The model under review builds one solid part; all positions refer to its coordinate system, in mm. A direction names the side the tool comes from. Round coordinates to 2 decimals unless told otherwise and drop trailing zeros. Order: outer loops, then holes, each group sorted by start corner. A loop starts at its lowest first (then second) coordinate and runs counter-clockwise, first axis right, second up.
from build123d import *

# Parameters (mm, degrees)
SKETCH_1_W                         = 50
SKETCH_1_H                         = 80
SM_BASE_FLANGE_1_DEPTH             = 3
SM_EDGE_FLANGE_1_STRIP_W           = 13.4732
SM_EDGE_FLANGE_1_STRIP_H           = 3
SM_EDGE_FLANGE_1_STRIP_CUT_DEPTH   = 50
SM_EDGE_FLANGE_1_STRIP_2_W         = 13.4732
SM_EDGE_FLANGE_1_STRIP_2_H         = 3
SM_EDGE_FLANGE_1_STRIP_CUT_2_DEPTH = 50
SM_EDGE_FLANGE_1_DEPTH             = 50
SM_EDGE_FLANGE_1_BEND_DEPTH        = 50
SM_EDGE_FLANGE_2_STRIP_W           = 13.4732
SM_EDGE_FLANGE_2_STRIP_H           = 3
SM_EDGE_FLANGE_2_STRIP_CUT_DEPTH   = 50
SM_EDGE_FLANGE_2_STRIP_2_W         = 13.4732
SM_EDGE_FLANGE_2_STRIP_2_H         = 3
SM_EDGE_FLANGE_2_STRIP_CUT_2_DEPTH = 50
SM_EDGE_FLANGE_2_DEPTH             = 50
SM_EDGE_FLANGE_2_BEND_DEPTH        = 50
SKETCH_18_R                        = 6.5
CUT_EXTRUDE_1_DEPTH                = 124


# Sheet-metal steps are written as plain solids
with BuildPart() as part:
    # Sketch 1 → 基体-法兰1 (new body)
    with BuildSketch(Plane.XY):
        with Locations((25, 40)):
            Rectangle(SKETCH_1_W, SKETCH_1_H)
    extrude(amount=-SM_BASE_FLANGE_1_DEPTH)

    # 边线-法兰1 strip (across the edge) → 边线-法兰1 strip cut (cut)
    with BuildSketch(Plane(origin=(0, 80, -3), x_dir=(0, -1, 0), z_dir=(1, 0, 0))):
        with Locations((-6, -1.5)):
            Rectangle(SM_EDGE_FLANGE_1_STRIP_W, SM_EDGE_FLANGE_1_STRIP_H)
    extrude(amount=SM_EDGE_FLANGE_1_STRIP_CUT_DEPTH, mode=Mode.SUBTRACT)

    # 边线-法兰1 strip 2 (across the edge) → 边线-法兰1 strip cut 2 (cut)
    with BuildSketch(Plane(origin=(50, 0, -3), x_dir=(0, 1, 0), z_dir=(-1, 0, 0))):
        with Locations((-6, -1.5)):
            Rectangle(SM_EDGE_FLANGE_1_STRIP_2_W, SM_EDGE_FLANGE_1_STRIP_2_H)
    extrude(amount=SM_EDGE_FLANGE_1_STRIP_CUT_2_DEPTH, mode=Mode.SUBTRACT)

    # 边线-法兰1 section (across the edge) → 边线-法兰1 (add)
    with BuildSketch(Plane(origin=(0, 80, -3), x_dir=(0, -1, 0), z_dir=(1, 0, 0))):
        with BuildLine():
            Line((-3, 0.7366), (-3, 17))
            Line((-3, 17), (0, 17))
            Line((0, 17), (0, 0.7366))
            ThreePointArc((0, 0.7366), (0.215745145, 0.215745145), (0.7366, 0))
            Line((0.7366, 0), (0.7366, -3))
            ThreePointArc((0.7366, -3), (-1.905575199, -1.905575199), (-3, 0.7366))
        make_face()
    extrude(amount=SM_EDGE_FLANGE_1_DEPTH)

    # 边线-法兰1 section 2 (across the edge) → 边线-法兰1 bend (add)
    with BuildSketch(Plane(origin=(50, 0, -3), x_dir=(0, 1, 0), z_dir=(-1, 0, 0))):
        with BuildLine():
            Line((-3, 0.7366), (-3, 17))
            Line((-3, 17), (0, 17))
            Line((0, 17), (0, 0.7366))
            ThreePointArc((0, 0.7366), (0.215745145, 0.215745145), (0.7366, 0))
            Line((0.7366, 0), (0.7366, -3))
            ThreePointArc((0.7366, -3), (-1.905575199, -1.905575199), (-3, 0.7366))
        make_face()
    extrude(amount=SM_EDGE_FLANGE_1_BEND_DEPTH)

    # 边线-法兰2 strip (across the edge) → 边线-法兰2 strip cut (cut)
    with BuildSketch(Plane(origin=(0, -3, -20), x_dir=(0, 0, 1), z_dir=(1, 0, 0))):
        with Locations((-6, -1.5)):
            Rectangle(SM_EDGE_FLANGE_2_STRIP_W, SM_EDGE_FLANGE_2_STRIP_H)
    extrude(amount=SM_EDGE_FLANGE_2_STRIP_CUT_DEPTH, mode=Mode.SUBTRACT)

    # 边线-法兰2 strip 2 (across the edge) → 边线-法兰2 strip cut 2 (cut)
    with BuildSketch(Plane(origin=(50, 83, -20), x_dir=(0, 0, 1), z_dir=(-1, 0, 0))):
        with Locations((-6, -1.5)):
            Rectangle(SM_EDGE_FLANGE_2_STRIP_2_W, SM_EDGE_FLANGE_2_STRIP_2_H)
    extrude(amount=SM_EDGE_FLANGE_2_STRIP_CUT_2_DEPTH, mode=Mode.SUBTRACT)

    # 边线-法兰2 section (across the edge) → 边线-法兰2 (add)
    with BuildSketch(Plane(origin=(0, -3, -20), x_dir=(0, 0, 1), z_dir=(1, 0, 0))):
        with BuildLine():
            Line((-3, 0.7366), (-3, 27))
            Line((-3, 27), (0, 27))
            Line((0, 27), (0, 0.7366))
            ThreePointArc((0, 0.7366), (0.215745145, 0.215745145), (0.7366, 0))
            Line((0.7366, 0), (0.7366, -3))
            ThreePointArc((0.7366, -3), (-1.905575199, -1.905575199), (-3, 0.7366))
        make_face()
    extrude(amount=SM_EDGE_FLANGE_2_DEPTH)

    # 边线-法兰2 section 2 (across the edge) → 边线-法兰2 bend (add)
    with BuildSketch(Plane(origin=(50, 83, -20), x_dir=(0, 0, 1), z_dir=(-1, 0, 0))):
        with BuildLine():
            Line((-3, 0.7366), (-3, 27))
            Line((-3, 27), (0, 27))
            Line((0, 27), (0, 0.7366))
            ThreePointArc((0, 0.7366), (0.215745145, 0.215745145), (0.7366, 0))
            Line((0.7366, 0), (0.7366, -3))
            ThreePointArc((0.7366, -3), (-1.905575199, -1.905575199), (-3, 0.7366))
        make_face()
    extrude(amount=SM_EDGE_FLANGE_2_BEND_DEPTH)

    # 草图18 → 切除-拉伸1 (cut, through all)
    with BuildSketch(Plane.XY):
        with Locations((25, 40)):
            Circle(SKETCH_18_R)
    extrude(amount=-CUT_EXTRUDE_1_DEPTH, mode=Mode.SUBTRACT)


solid = part.part
(1) To check wall thickness, follow L1, parallel to Y at x = 11.5, z = -15.5; L2, parallel to Z at x = 36.5, y = 6; L3, parallel to Z at x = 34.5, y = 91. State the ranges of each line that lie inside material, in increasing order.
(2) Tool access review of faces 1 (the flat face through (25, 83, -11)), 2 (the cylindrical face through (25.35, 81.07, -21.88)), 3 (the flat face through (25, 49, 0)): name each direction out of +Z, -Z, +X, -X, +Y, -Y from which nothing blocks a thin tool from reaching the whole face with its end or side.
(3) The part is to be moulded in two halves that separate along Y. For faces 4 (the flat face through (25, 110, -22)), 5 (the cylindrical face through (19.842, 36.045, -1.479)), 6 (the flat face through (25, -3, -11)), say which applies: pulls with the +Y half, pulls with the -Y half, needs draft (parallel to the pull), parting line crosses it, or undercut.
(4) We need section B-B (z = -10.5). Give the boundary of the cut face in (x, y), and give its area (3 significant figures).
(5) Clearance check with flat-ended pins moving along their axes: P1, Ø1.5, axis at x = 41, z = -13.5, coming from the -Y side; P2, Ø12.5, axis at x = 26, z = -14, coming from the +Y side; P3, Ø8, axis at x = 32, y = 22, coming from the -Z side; P4, Ø8, axis at x = 30.5, y = -21, coming from the +Z side. State where each tip first meets the part, or that it passes through.
(6) We need section C-C (y = 40). Give the boundary of the cut face in (x, z), and give its area (3 significant figures).
(7) We need section A-A (x = 25). Give the boundary of the cut face in (y, z), and give its area (3 significant figures).
(8) We need section D-D (x = 35.5). Give the boundary of the cut face in (y, z), and give its area (3 significant figures).
Verdict:
1. L1: y = -3 to 0, 80 to 83
1. L2: z = -3 to 0
1. L3: z = -23 to -20
2. face 1: +Z, +X, -X, +Y
2. face 2: -Z, +X, -X
2. face 3: +Z, +X, -X, +Y, -Y
3. face 4: pulls with the +Y half
3. face 5: undercut
3. face 6: pulls with the -Y half
4. outline: (0, -3) - (50, -3) - (50, 0) - (0, 0) - close; (0, 80) - (50, 80) - (50, 83) - (0, 83) - close
4. area: 300 mm2
5. P1: stops at y = -3
5. P2: stops at y = 110
5. P3: stops at z = -3
5. P4: stops at z = -20
6. outline: (0, -3) - (18.5, -3) - (18.5, 0) - (0, 0) - close; (31.5, -3) - (50, -3) - (50, 0) - (31.5, 0) - close
6. area: 111 mm2
7. outline: (-30, -23) - (-3.74, -23) arc R3.74 ccw to (0, -19.26) - (0, -3.74) arc R0.74 cw to (0.74, -3) - (33.5, -3) - (33.5, 0) - (0.74, 0) arc R3.74 ccw to (-3, -3.74) - (-3, -19.26) arc R0.74 cw to (-3.74, -20) - (-30, -20) - close; (46.5, -3) - (79.26, -3) arc R0.74 cw to (80, -3.74) - (80, -19.26) arc R3.74 ccw to (83.74, -23) - (110, -23) - (110, -20) - (83.74, -20) arc R0.74 cw to (83, -19.26) - (83, -3.74) arc R3.74 ccw to (79.26, 0) - (46.5, 0) - close
7. area: 489 mm2
8. outline: (-30, -23) - (-3.74, -23) arc R3.74 ccw to (0, -19.26) - (0, -3.74) arc R0.74 cw to (0.74, -3) - (79.26, -3) arc R0.74 cw to (80, -3.74) - (80, -19.26) arc R3.74 ccw to (83.74, -23) - (110, -23) - (110, -20) - (83.74, -20) arc R0.74 cw to (83, -19.26) - (83, -3.74) arc R3.74 ccw to (79.26, 0) - (0.74, 0) arc R3.74 ccw to (-3, -3.74) - (-3, -19.26) arc R0.74 cw to (-3.74, -20) - (-30, -20) - close
8. area: 528 mm2
